Here's the drawing with two shaded views (mm, measured from the low corner). I have some questions. Round coordinates to 2 decimals unless told otherwise and drop trailing zeros. Loops run counter-clockwise (first coordinate to the right, second up) from the corner with the lowest first, then second, coordinate; pieces in that order, holes last. Notation, with made-up numbers: (66, 66) -> (95, 66) arc R32 ccw to (95, 103) -> close; hole circle Ø6 at (-29, 3). An arc over 180 degrees is marked (long way). One line per item, written item: value. Start each with the question number.
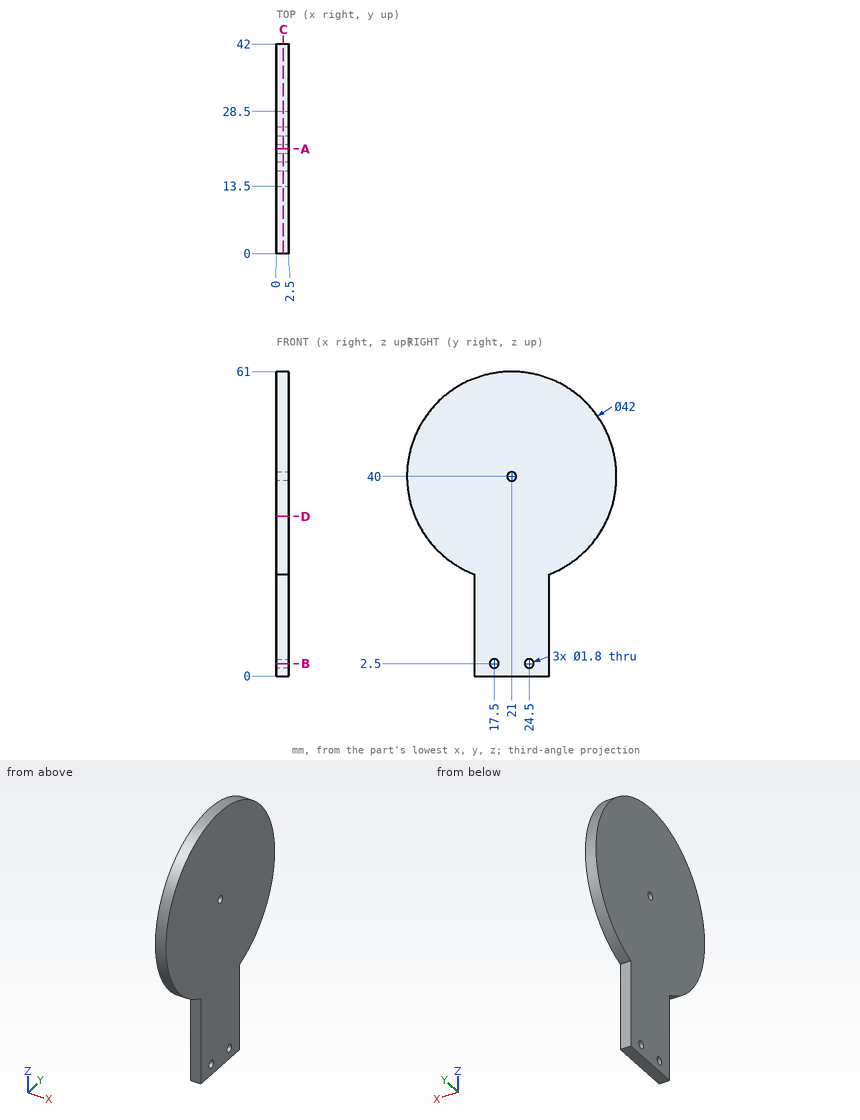
Q1. I want a section at B-B on z = 2.5. Please give me the cut outline in (x, y).
Q2. I want a section at A-A on y = 21. Please give me the cut outline in (x, z), plus the area to 3 significant figures.
Q3. I want a section at D-D on z = 32. Please give me the cut outline in (x, y), plus the area to 3 significant figures.
Q4. If I drill on line 1 along Y through (x, z) = (0.85, 2.5); line 2 along Y through (x, z) = (1.55, 40); line 3 along Y through (x, z) = (0.1, 3.5), over which ranges is the centre line in solid material (lowest first)?
Q5. I want a section at C-C on x = 1.4. Please give me the cut outline in (y, z).
Q6. Will this pin go through, and if not, where does the flat tip stop? P1, Ø1, axis at x = 2, z = 10, coming from the +Y side.
Answers below:
1. outline: (0, 13.5) -> (2.5, 13.5) -> (2.5, 16.6) -> (0, 16.6) -> close; (0, 18.4) -> (2.5, 18.4) -> (2.5, 23.6) -> (0, 23.6) -> close; (0, 25.4) -> (2.5, 25.4) -> (2.5, 28.5) -> (0, 28.5) -> close
2. outline: (0, 0) -> (2.5, 0) -> (2.5, 39.1) -> (0, 39.1) -> close; (0, 40.9) -> (2.5, 40.9) -> (2.5, 61) -> (0, 61) -> close
2. area: 148 mm^2
3. outline: (0, 1.58) -> (2.5, 1.58) -> (2.5, 40.42) -> (0, 40.42) -> close
3. area: 97.1 mm^2
4. line 1: y = 13.5 to 16.6, 18.4 to 23.6, 25.4 to 28.5
4. line 2: y = 0 to 20.1, 21.9 to 42
4. line 3: y = 13.5 to 28.5
5. outline: (13.5, 0) -> (28.5, 0) -> (28.5, 20.38) arc R21 ccw (long way) to (13.5, 20.38) -> close; hole circle Ø1.8 at (17.5, 2.5); hole circle Ø1.8 at (21, 40); hole circle Ø1.8 at (24.5, 2.5)
6. P1: stops at y = 28.5
